The listing builds one solid part. Answer for the finished solid, in the listing's coordinates (mm). Give positions to 0.01 mm unless a question says otherwise; leave off trailing zeros. Loops run counter-clockwise (first coordinate to the right, second up) from the corner with the lowest first, then second, coordinate; pieces in that order, holes last.
Item 1: Each of these flat-tipped pins is pushed along its axis until it touches: pin 1 Ø1 at (x, z) = (-17.5, -39) entering from -Y; pin 2 Ø3.5 at (x, y) = (48.5, 1.5) entering from -Z; pin 3 Ø2.5 at (x, z) = (17.75, -96.7) entering from +Y; pin 4 Ø0.9 at (y, z) = (2, -103.5) entering from -X. Where does it stop, or does it pass through?
Item 2: Section B-B, the plane y = 6.5 is taken. Give the number of separate pieces and of enclosed holes in the cut face, and give its area (3 significant figures).
Item 3: Section C-C, the plane z = -35 is taken. Give the vertices of the cut face in (x, y), and give its area (3 significant figures).
Item 4: Consider line 1 along X through (y, z) = (6, -50.5); line 2 along Z through (x, y) = (16, 6.25); line 3 along X through (y, z) = (6.25, -4). Determine where each line is inside the solid, lowest interval first.
Item 5: Section A-A, the plane x = -61 is taken. Give the vertices of the cut face in (y, z), and give its area (3 significant figures).
Item 6: Section D-D, the plane z = 12 is taken. Give the vertices of the cut face in (x, y).
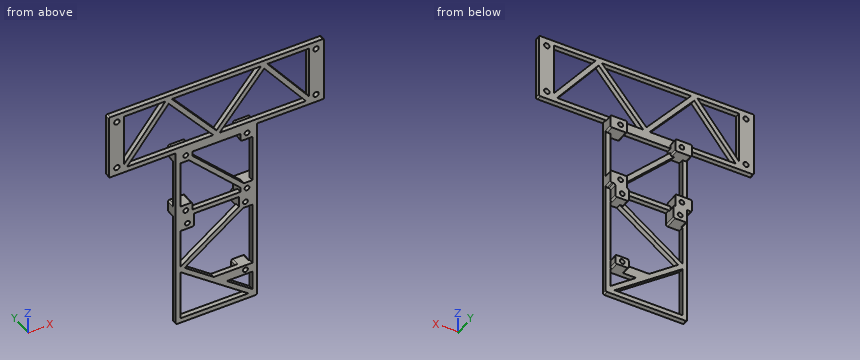
from build123d import *

# Parameters (mm, degrees)
SKETCH1_R           = 1.65
SKETCH1_W           = 29.5
SKETCH1_H           = 3
SKETCH1_R_2         = 1.5
SKETCH1_W_2         = 3
SKETCH1_H_2         = 29.5
SKETCH1_H_3         = 8.6
SKETCH1_W_3         = 8.25
SKETCH1_H_4         = 6
SKETCH1_H_5         = 1.5
BOSS_EXTRUDE1_DEPTH = 3
BOSS_EXTRUDE2_START = 3
SKETCH1_5_R         = 1.5
SKETCH1_5_W         = 8.25
SKETCH1_5_H         = 6
BOSS_EXTRUDE2_DEPTH = 5
FILLET1_R           = 1


with BuildPart() as part:
    # Sketch1 → Boss-Extrude1 (new body)
    # profile 1 of 27: a face of its own
    with BuildSketch(Plane(origin=(0, 0, 0), x_dir=(1, 0, 0), z_dir=(0, 1, 0))):
        Polygon((-56.65, -37.9), (-56.65, -40.9), (56.65, -40.9), (56.65, -37.9), (31.205729157, -37.9), (27.341462913, -37.9), (-27.341462913, -37.9), (-31.205729157, -37.9), align=None)
    # profile 2 of 27: a face of its own
    with BuildSketch(Plane(origin=(0, 0, 0), x_dir=(1, 0, 0), z_dir=(0, 1, 0))):
        Polygon((-65.95, 0), (-65.95, -40.9), (-56.65, -40.9), (-56.65, -37.9), (-56.65, -5.431807955), (-56.65, -3), (-56.65, 0), align=None)
        with Locations(Location((-61, -35.95, 0), (0, 0, 270))):
            Circle(SKETCH1_R, mode=Mode.SUBTRACT)
        with Locations(Location((-61, -4.95, 0), (0, 0, 270))):
            Circle(SKETCH1_R, mode=Mode.SUBTRACT)
    # profile 3 of 27: a face of its own
    with BuildSketch(Plane(origin=(0, 0, 0), x_dir=(1, 0, 0), z_dir=(0, 1, 0))):
        Polygon((-56.65, -3), (-56.65, -5.431807955), (-31.205729157, -37.9), (-27.341462913, -37.9), (0, -5.332864995), (27.341462913, -37.9), (31.205729157, -37.9), (56.65, -5.431807955), (56.65, -3), (54.744270843, -3), (29.259896294, -35.519366427), (1.958537087, -3), (-1.958537087, -3), (-29.259896294, -35.519366427), (-54.744270843, -3), align=None)
    # profile 4 of 27: a face of its own
    with BuildSketch(Plane(origin=(0, 0, 0), x_dir=(1, 0, 0), z_dir=(0, 1, 0))):
        Polygon((56.65, -37.9), (56.65, -40.9), (65.95, -40.9), (65.95, 0), (56.65, 0), (56.65, -3), (56.65, -5.431807955), align=None)
        with Locations(Location((61, -35.95, 0), (0, 0, 270))):
            Circle(SKETCH1_R, mode=Mode.SUBTRACT)
        with Locations(Location((61, -4.95, 0), (0, 0, 270))):
            Circle(SKETCH1_R, mode=Mode.SUBTRACT)
    # profile 5 of 27: a face of its own
    with BuildSketch(Plane(origin=(0, 0, 0), x_dir=(1, 0, 0), z_dir=(0, 1, 0))):
        Polygon((-25, 0), (-56.65, 0), (-56.65, -3), (-54.744270843, -3), (-1.958537087, -3), (1.958537087, -3), (54.744270843, -3), (56.65, -3), (56.65, 0), (25, 0), (14.75, 0), (-14.75, 0), align=None)
    # profile 6 of 27: a face of its own
    with BuildSketch(Plane(origin=(0, 0, 0), x_dir=(1, 0, 0), z_dir=(0, 1, 0))):
        with Locations((0, 1.5)):
            Rectangle(SKETCH1_W, SKETCH1_H)
    # profile 7 of 27: a face of its own
    with BuildSketch(Plane(origin=(0, 0, 0), x_dir=(1, 0, 0), z_dir=(0, 1, 0))):
        Polygon((14.75, 3), (14.75, 0), (25, 0), (25, 8), (22, 8), (14.75, 8), align=None)
        with Locations(Location((18.75, 4, 0), (0, 0, 270))):
            Circle(SKETCH1_R_2, mode=Mode.SUBTRACT)
    # profile 8 of 27: a face of its own
    with BuildSketch(Plane(origin=(0, 0, 0), x_dir=(1, 0, 0), z_dir=(0, 1, 0))):
        Polygon((-25, 8), (-25, 0), (-14.75, 0), (-14.75, 3), (-14.75, 5.878679656), (-14.75, 8), (-16.871320344, 8), (-22, 8), align=None)
        with Locations(Location((-18.75, 4, 0), (0, 0, 270))):
            Circle(SKETCH1_R_2, mode=Mode.SUBTRACT)
    # profile 9 of 27: a face of its own
    with BuildSketch(Plane(origin=(0, 0, 0), x_dir=(1, 0, 0), z_dir=(0, 1, 0))):
        with Locations((23.5, 22.75)):
            Rectangle(SKETCH1_W_2, SKETCH1_H_2)
    # profile 10 of 27: a face of its own
    with BuildSketch(Plane(origin=(0, 0, 0), x_dir=(1, 0, 0), z_dir=(0, 1, 0))):
        Polygon((-14.75, 8), (-14.75, 5.878679656), (16.871320344, 37.5), (14.75, 37.5), (14.75, 39.621320344), (-16.871320344, 8), align=None)
    # profile 11 of 27: a face of its own
    with BuildSketch(Plane(origin=(0, 0, 0), x_dir=(1, 0, 0), z_dir=(0, 1, 0))):
        with Locations((-23.5, 22.75)):
            Rectangle(SKETCH1_W_2, SKETCH1_H_2)
    # profile 12 of 27: a face of its own
    with BuildSketch(Plane(origin=(0, 0, 0), x_dir=(1, 0, 0), z_dir=(0, 1, 0))):
        Polygon((14.75, 37.5), (16.871320344, 37.5), (22, 37.5), (25, 37.5), (25, 45.5), (22, 45.5), (14.75, 45.5), (14.75, 42.5), (14.75, 39.621320344), align=None)
        with Locations(Location((18.75, 41.5, 0), (0, 0, 270))):
            Circle(SKETCH1_R_2, mode=Mode.SUBTRACT)
    # profile 13 of 27: a face of its own
    with BuildSketch(Plane(origin=(0, 0, 0), x_dir=(1, 0, 0), z_dir=(0, 1, 0))):
        Polygon((-13.75, 45.5), (-14.75, 45.5), (-14.75, 42.5), (14.75, 42.5), (14.75, 45.5), (13.75, 45.5), align=None)
    # profile 14 of 27: a face of its own
    with BuildSketch(Plane(origin=(0, 0, 0), x_dir=(1, 0, 0), z_dir=(0, 1, 0))):
        Polygon((-25, 45.5), (-25, 37.5), (-22, 37.5), (-14.75, 37.5), (-14.75, 42.5), (-14.75, 45.5), (-22, 45.5), align=None)
        with Locations(Location((-18.75, 41.5, 0), (0, 0, 270))):
            Circle(SKETCH1_R_2, mode=Mode.SUBTRACT)
    # profile 15 of 27: a face of its own
    with BuildSketch(Plane(origin=(0, 0, 0), x_dir=(1, 0, 0), z_dir=(0, 1, 0))):
        Polygon((-22, 54.1), (-22, 45.5), (-14.75, 45.5), (-13.75, 45.5), (-13.75, 54.1), align=None)
        with Locations(Location((-17.75, 50.5, 0), (0, 0, 270))):
            Circle(SKETCH1_R_2, mode=Mode.SUBTRACT)
    # profile 16 of 27: a face of its own
    with BuildSketch(Plane(origin=(0, 0, 0), x_dir=(1, 0, 0), z_dir=(0, 1, 0))):
        with Locations((-23.5, 49.8)):
            Rectangle(SKETCH1_W_2, SKETCH1_H_3)
    # profile 17 of 27: a face of its own
    with BuildSketch(Plane(origin=(0, 0, 0), x_dir=(1, 0, 0), z_dir=(0, 1, 0))):
        Polygon((13.75, 45.5), (14.75, 45.5), (22, 45.5), (22, 54.1), (16.290717268, 54.1), (13.75, 54.1), (13.75, 52.241545271), align=None)
        with Locations(Location((17.75, 50.5, 0), (0, 0, 270))):
            Circle(SKETCH1_R_2, mode=Mode.SUBTRACT)
    # profile 18 of 27: a face of its own
    with BuildSketch(Plane(origin=(0, 0, 0), x_dir=(1, 0, 0), z_dir=(0, 1, 0))):
        with Locations((23.5, 49.8)):
            Rectangle(SKETCH1_W_2, SKETCH1_H_3)
    # profile 19 of 27: a face of its own
    with BuildSketch(Plane(origin=(0, 0, 0), x_dir=(1, 0, 0), z_dir=(0, 1, 0))):
        Polygon((-22, 82.130125999), (-22, 78.391545271), (13.75, 52.241545271), (13.75, 54.1), (16.290717268, 54.1), (-19.459282732, 80.25), (-1.660786492, 93.7), (6.279063132, 99.7), (22, 111.580026156), (22, 113.5), (19.512013715, 113.5), align=None)
    # profile 20 of 27: a face of its own
    with BuildSketch(Plane(origin=(0, 0, 0), x_dir=(1, 0, 0), z_dir=(0, 1, 0))):
        Polygon((22, 54.1), (25, 54.1), (25, 113.5), (22, 113.5), (22, 111.580026156), (22, 99.7), (22, 93.7), align=None)
    # profile 21 of 27: a face of its own
    with BuildSketch(Plane(origin=(0, 0, 0), x_dir=(1, 0, 0), z_dir=(0, 1, 0))):
        Polygon((-25, 113.5), (-25, 54.1), (-22, 54.1), (-22, 78.391545271), (-22, 82.130125999), (-22, 113.5), align=None)
    # profile 22 of 27: a face of its own
    with BuildSketch(Plane(origin=(0, 0, 0), x_dir=(1, 0, 0), z_dir=(0, 1, 0))):
        Polygon((-1.660786492, 93.7), (13.75, 93.7), (13.75, 99.7), (6.279063132, 99.7), align=None)
    # profile 23 of 27: a face of its own
    with BuildSketch(Plane(origin=(0, 0, 0), x_dir=(1, 0, 0), z_dir=(0, 1, 0))):
        with Locations((17.875, 96.7)):
            Rectangle(SKETCH1_W_3, SKETCH1_H_4)
        with Locations(Location((17.75, 96.7, 0), (0, 0, 270))):
            Circle(SKETCH1_R_2, mode=Mode.SUBTRACT)
    # profile 24 of 27: a face of its own
    with BuildSketch(Plane(origin=(0, 0, 0), x_dir=(1, 0, 0), z_dir=(0, 1, 0))):
        Polygon((-22, 115), (-22, 113.5), (19.512013715, 113.5), (22, 113.5), (22, 115), align=None)
    # profile 25 of 27: a face of its own
    with BuildSketch(Plane(origin=(0, 0, 0), x_dir=(1, 0, 0), z_dir=(0, 1, 0))):
        Polygon((-25, 116.5), (-25, 115), (-22, 115), (22, 115), (25, 115), (25, 116.5), align=None)
    # profile 26 of 27: a face of its own
    with BuildSketch(Plane(origin=(0, 0, 0), x_dir=(1, 0, 0), z_dir=(0, 1, 0))):
        with Locations((23.5, 114.25)):
            Rectangle(SKETCH1_W_2, SKETCH1_H_5)
    # profile 27 of 27: a face of its own
    with BuildSketch(Plane(origin=(0, 0, 0), x_dir=(1, 0, 0), z_dir=(0, 1, 0))):
        with Locations((-23.5, 114.25)):
            Rectangle(SKETCH1_W_2, SKETCH1_H_5)
    extrude(amount=BOSS_EXTRUDE1_DEPTH)

    # Sketch1<5> → Boss-Extrude2 (add)
    # profile 1 of 7: a face of its own
    with BuildSketch(Plane(origin=(0, 0, 0), x_dir=(1, 0, 0), z_dir=(0, 1, 0)).offset(BOSS_EXTRUDE2_START)):
        Polygon((14.75, 3), (14.75, 0), (25, 0), (25, 8), (22, 8), (14.75, 8), align=None)
        with Locations(Location((18.75, 4, 0), (0, 0, 270))):
            Circle(SKETCH1_5_R, mode=Mode.SUBTRACT)
    # profile 2 of 7: a face of its own
    with BuildSketch(Plane(origin=(0, 0, 0), x_dir=(1, 0, 0), z_dir=(0, 1, 0)).offset(BOSS_EXTRUDE2_START)):
        Polygon((-25, 8), (-25, 0), (-14.75, 0), (-14.75, 3), (-14.75, 5.878679656), (-14.75, 8), (-16.871320344, 8), (-22, 8), align=None)
        with Locations(Location((-18.75, 4, 0), (0, 0, 270))):
            Circle(SKETCH1_5_R, mode=Mode.SUBTRACT)
    # profile 3 of 7: a face of its own
    with BuildSketch(Plane(origin=(0, 0, 0), x_dir=(1, 0, 0), z_dir=(0, 1, 0)).offset(BOSS_EXTRUDE2_START)):
        Polygon((14.75, 37.5), (16.871320344, 37.5), (22, 37.5), (25, 37.5), (25, 45.5), (22, 45.5), (14.75, 45.5), (14.75, 42.5), (14.75, 39.621320344), align=None)
        with Locations(Location((18.75, 41.5, 0), (0, 0, 270))):
            Circle(SKETCH1_5_R, mode=Mode.SUBTRACT)
    # profile 4 of 7: a face of its own
    with BuildSketch(Plane(origin=(0, 0, 0), x_dir=(1, 0, 0), z_dir=(0, 1, 0)).offset(BOSS_EXTRUDE2_START)):
        Polygon((-25, 45.5), (-25, 37.5), (-22, 37.5), (-14.75, 37.5), (-14.75, 42.5), (-14.75, 45.5), (-22, 45.5), align=None)
        with Locations(Location((-18.75, 41.5, 0), (0, 0, 270))):
            Circle(SKETCH1_5_R, mode=Mode.SUBTRACT)
    # profile 5 of 7: a face of its own
    with BuildSketch(Plane(origin=(0, 0, 0), x_dir=(1, 0, 0), z_dir=(0, 1, 0)).offset(BOSS_EXTRUDE2_START)):
        Polygon((13.75, 45.5), (14.75, 45.5), (22, 45.5), (22, 54.1), (16.290717268, 54.1), (13.75, 54.1), (13.75, 52.241545271), align=None)
        with Locations(Location((17.75, 50.5, 0), (0, 0, 270))):
            Circle(SKETCH1_5_R, mode=Mode.SUBTRACT)
    # profile 6 of 7: a face of its own
    with BuildSketch(Plane(origin=(0, 0, 0), x_dir=(1, 0, 0), z_dir=(0, 1, 0)).offset(BOSS_EXTRUDE2_START)):
        Polygon((-22, 54.1), (-22, 45.5), (-14.75, 45.5), (-13.75, 45.5), (-13.75, 54.1), align=None)
        with Locations(Location((-17.75, 50.5, 0), (0, 0, 270))):
            Circle(SKETCH1_5_R, mode=Mode.SUBTRACT)
    # profile 7 of 7: a face of its own
    with BuildSketch(Plane(origin=(0, 0, 0), x_dir=(1, 0, 0), z_dir=(0, 1, 0)).offset(BOSS_EXTRUDE2_START)):
        with Locations((17.875, 96.7)):
            Rectangle(SKETCH1_5_W, SKETCH1_5_H)
        with Locations(Location((17.75, 96.7, 0), (0, 0, 270))):
            Circle(SKETCH1_5_R, mode=Mode.SUBTRACT)
    extrude(amount=BOSS_EXTRUDE2_DEPTH)

    # Fillet1
    fillet1_edges = [part.edges().sort_by_distance(p)[0] for p in [
        (14.75, 4, -8),
        (-14.75, 4, -37.5),
        (-13.75, 4, -54.1),
        (65.95, 1.5, 0),
        (65.95, 1.5, 40.9),
        (-65.95, 1.5, 40.9),
        (-65.95, 1.5, 0),
        (-25, 1.5, -116.5),
        (25, 1.5, -116.5),
        (14.75, 5.5, 0),
        (25, 5.5, 0),
        (25, 5.5, -8),
        (-25, 5.5, -8),
        (-25, 5.5, 0),
        (-14.75, 5.5, 0),
        (-14.75, 5.5, -8),
        (13.75, 5.5, -45.5),
        (14.75, 5.5, -37.5),
        (25, 5.5, -37.5),
        (25, 5.5, -45.5),
        (22, 5.5, -45.5),
        (22, 5.5, -54.1),
        (13.75, 5.5, -54.1),
        (-13.75, 5.5, -45.5),
        (-22, 5.5, -54.1),
        (-25, 5.5, -45.5),
        (-25, 5.5, -37.5),
        (13.75, 5.5, -93.7),
        (22, 5.5, -93.7),
        (22, 5.5, -99.7),
        (13.75, 5.5, -99.7),
    ]]
    fillet(fillet1_edges, radius=FILLET1_R - 0.0001)  # a hair under: the kernel refuses the full size


solid = part.part
Worked answers:
1. pin 1: stops at y = 0
1. pin 2: stops at z = 0
1. pin 3: passes through
1. pin 4: stops at x = -25
2. separate pieces: 5
2. enclosed holes: 7
2. area: 465 mm2
3. outline: (-25, 0) - (-22, 0) - (-22, 3) - (-25, 3) - close; (10.13, 0) - (14.37, 0) - (14.37, 3) - (10.13, 3) - close; (22, 0) - (25, 0) - (25, 3) - (22, 3) - close
3. area: 30.7 mm2
4. line 1: x = -22 to -19.25, -16.25 to -13.75, 13.75 to 16.25, 19.25 to 22
4. line 2: z = -99.7 to -93.7, -54.1 to -37.5, -8 to 0
4. line 3: x = -25 to -20.25, -17.25 to -14.75, 14.75 to 17.25, 20.25 to 25
5. outline: (0, 0) - (3, 0) - (3, 3.3) - (0, 3.3) - close; (0, 6.6) - (3, 6.6) - (3, 34.3) - (0, 34.3) - close; (0, 37.6) - (3, 37.6) - (3, 40.9) - (0, 40.9) - close
5. area: 103 mm2
6. outline: (-65.95, 0) - (-56.65, 0) - (-56.65, 3) - (-65.95, 3) - close; (-51.5, 0) - (-47.69, 0) - (-47.69, 3) - (-51.5, 3) - close; (-9.51, 0) - (-5.6, 0) - (-5.6, 3) - (-9.51, 3) - close; (5.6, 0) - (9.51, 0) - (9.51, 3) - (5.6, 3) - close; (47.69, 0) - (51.5, 0) - (51.5, 3) - (47.69, 3) - close; (56.65, 0) - (65.95, 0) - (65.95, 3) - (56.65, 3) - close
